```python
from build123d import *

# Parameters (mm, degrees)
F0_R     = 2
F1_DEPTH = 3


with BuildPart() as f1:
    # F0 (on Top) → F1 (new body)
    with BuildSketch(Plane.XY):
        with BuildLine():
            Line((-35.222202, 0), (0, 0))
            Line((0, 0), (35.222202, 0))
            ThreePointArc((35.222202, 0), (37.742959, 0.555205), (39.797202, 2.118071))
            Line((39.797202, 2.118071), (62.454529, 28.820584))
            ThreePointArc((62.454529, 28.820584), (63.512024, 30.634906), (63.879529, 32.702513))
            Line((63.879529, 32.702513), (63.879529, 42))
            ThreePointArc((63.879529, 42), (63.000849, 44.12132), (60.879529, 45))
            Line((60.879529, 45), (45.493925, 45))
            ThreePointArc((45.493925, 45), (44.0723, 44.641777), (42.990182, 43.652656))
            Line((42.990182, 43.652656), (41.424434, 41.280578))
            ThreePointArc((41.424434, 41.280578), (40.443151, 40.137329), (39.208001, 39.274578))
            Line((39.208001, 39.274578), (36.484002, 37.843138))
            ThreePointArc((36.484002, 37.843138), (35.311788, 36.738841), (34.879529, 35.187483))
            Line((34.879529, 35.187483), (34.879529, 20))
            ThreePointArc((34.879529, 20), (33.122169, 15.757359), (28.879529, 14))
            Line((28.879529, 14), (0, 14))
            Line((0, 14), (-28.879529, 14))
            ThreePointArc((-28.879529, 14), (-33.122169, 15.757359), (-34.879529, 20))
            Line((-34.879529, 20), (-34.879529, 35.187483))
            ThreePointArc((-34.879529, 35.187483), (-35.311788, 36.738841), (-36.484002, 37.843138))
            Line((-36.484002, 37.843138), (-39.208001, 39.274578))
            ThreePointArc((-39.208001, 39.274578), (-40.443151, 40.137329), (-41.424434, 41.280578))
            Line((-41.424434, 41.280578), (-42.990182, 43.652656))
            ThreePointArc((-42.990182, 43.652656), (-44.0723, 44.641777), (-45.493925, 45))
            Line((-45.493925, 45), (-60.879529, 45))
            ThreePointArc((-60.879529, 45), (-63.000849, 44.12132), (-63.879529, 42))
            Line((-63.879529, 42), (-63.879529, 32.702513))
            ThreePointArc((-63.879529, 32.702513), (-63.512024, 30.634906), (-62.454529, 28.820584))
            Line((-62.454529, 28.820584), (-39.797202, 2.118071))
            ThreePointArc((-39.797202, 2.118071), (-37.742959, 0.555205), (-35.222202, 0))
        make_face()
        with Locations((-13, 8.5)):
            Circle(F0_R, mode=Mode.SUBTRACT)
        with Locations((13, 8.5)):
            Circle(F0_R, mode=Mode.SUBTRACT)
    extrude(amount=F1_DEPTH)


solid = f1.part
```
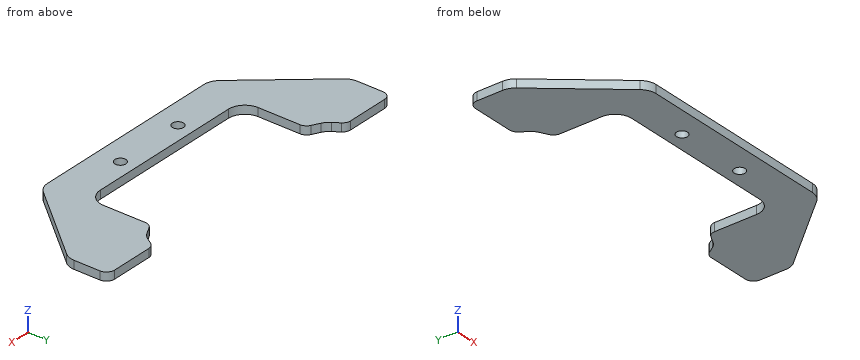
Can you work these out from the model? Positions are in its coordinate system, mm. Coordinates: 2 decimals unless noted, no trailing zeros. Loops run counter-clockwise (first coordinate to the right, second up) from the corner with the lowest first, then second, coordinate; pieces in that order, holes last. Notation, with made-up numbers: (26.5, 36.5) -> (83.5, 36.5) arc R13 cw to (83.5, 54.5) -> close; hole circle Ø11 at (-15.5, 17.5). An arc over 180 degrees is marked (long way). Put each result on its own line as item: value. Start each with the question number.
Q1. If I drill on line 1 (Y direction, x = -13, z = 2.35); line 2 (X direction, y = 38.5, z = 2.5); line 3 (X direction, y = 9, z = 1.9), over which ranges is the centre line in solid material (lowest first)? Write a range as [from, to].
Q2. I want a section at C-C (z = 2.2). Count the separate pieces of the cut face and the enclosed holes in it, plus the area to 3 significant figures.
Q3. I want a section at D-D (y = 8.5). Write out the boundary of the cut face in (x, z), plus the area to 3 significant figures.
Q4. I'm going to push flat-ended pins straight in: P1, Ø1.5, axis at y = 7.5, z = 2.5, coming from the +X side; P2, Ø0.9, axis at y = 25.5, z = 1, coming from the +X side; P3, Ø0.9, axis at x = -4.5, z = 2, coming from the +Y side. Where does each tip first touch, or does it pass through?
Q5. I want a section at A-A (x = -13). Write out the boundary of the cut face in (y, z).
Q6. I want a section at B-B (y = 17.5). Write out the boundary of the cut face in (x, z), plus the area to 3 significant figures.
Taken from the geometry:
1. line 1: y = [0, 6.5], [10.5, 14]
1. line 2: x = [-63.88, -37.73], [37.73, 63.88]
1. line 3: x = [-45.64, -14.94], [-11.06, 11.06], [14.94, 45.64]
2. separate pieces: 1
2. enclosed holes: 2
2. area: 2,690 mm2
3. outline: (-45.21, 0) -> (-15, 0) -> (-15, 3) -> (-45.21, 3) -> close; (-11, 0) -> (11, 0) -> (11, 3) -> (-11, 3) -> close; (15, 0) -> (45.21, 0) -> (45.21, 3) -> (15, 3) -> close
3. area: 247 mm2
4. P1: stops at x = 45
4. P2: stops at x = 60.02
4. P3: stops at y = 14
5. outline: (0, 0) -> (6.5, 0) -> (6.5, 3) -> (0, 3) -> close; (10.5, 0) -> (14, 0) -> (14, 3) -> (10.5, 3) -> close
6. outline: (-52.85, 0) -> (-34.33, 0) -> (-34.33, 3) -> (-52.85, 3) -> close; (34.33, 0) -> (52.85, 0) -> (52.85, 3) -> (34.33, 3) -> close
6. area: 111 mm2
